The model under review builds one solid part; all positions refer to its coordinate system, in mm. Coordinates: 2 decimals unless noted, no trailing zeros. Order: outer loops, then holes, each group sorted by start corner. A loop starts at its lowest first (then second) coordinate and runs counter-clockwise, first axis right, second up. Notation, with made-up numbers: (51, -33.75) -> (57, -33.75) arc R19 cw to (57, -17.75) -> close; hole circle Ø8 at (54, 23). An arc over 180 degrees is marked (long way). Use one line per item in the form item = value. Start each with the question number.
(1) Insertion check: pin 1 Ø0.7 at (x, z) = (-83.5, 39.5) entering from +Y; pin 2 Ø0.7 at (x, y) = (-84, -368) entering from +Z; pin 3 Ø1.5 at (x, z) = (-80, 2) entering from +Y. Each pin has a flat end and moves straight along its axis. Give the tip position at first contact, or say it passes through.
(2) Take a section at B-B (x = -76). State the section outline as (y, z) points.
(3) Mouldability with a two-part tool opening along Y and no side actions: class faces 1 (the flat face through (-83.342, -369, 46)), 2 (the flat face through (-79, -369, 85)), 3 (the cylindrical face through (-72.925, -367.02, 36.835)) as +Y half, -Y half, draft (parallel to the pull), parting line (faces both ways), or undercut.
(4) Wall thickness on line 1 along X through (y, z) = (-369, 50); line 2 along Y through (x, z) = (-78.75, 67); line 3 along Y through (x, z) = (-75.5, 54.5): over which ranges is each line inside the solid? List them lowest first.
(5) Take a section at A-A (y = -373). State the section outline as (x, z) points.
```python
from build123d import *

# Parameters (mm, degrees)
BOSS_EXTRUDE1_DEPTH      = 85
BOSS_EXTRUDE1_DEPTH_BACK = 10
SKETCH1_R                = 6
SKETCH2_W                = 2.203214475
SKETCH2_H                = 4.25945658
CUT_EXTRUDE1_DEPTH       = 80


with BuildPart() as part:
    # Sketch1 → Boss-Extrude1 (new, two sides: drawn at the far end of the back side and taken through both)
    with BuildSketch(Plane.XY.offset(-BOSS_EXTRUDE1_DEPTH_BACK)):
        with Locations((-78.64751379, -368.822211525)):
            Circle(SKETCH1_R)
    extrude(amount=BOSS_EXTRUDE1_DEPTH + BOSS_EXTRUDE1_DEPTH_BACK)

    # Sketch2 → Cut-Extrude1 (cut)
    with BuildSketch(Plane.XY.offset(85)):
        with Locations((-84.444038678, -368.822211525)):
            Rectangle(SKETCH2_W, SKETCH2_H)
    extrude(amount=-CUT_EXTRUDE1_DEPTH, mode=Mode.SUBTRACT)


solid = part.part
```
Findings:
q1.pin_1 = -364.86
q1.pin_2 = 5
q1.pin_3 = -362.85
q2.outline = (-374.21, -10) -> (-363.44, -10) -> (-363.44, 85) -> (-374.21, 85) -> close
q3.face_1 = undercut
q3.face_2 = draft
q3.face_3 = parting line
q4.line_1 = -83.34 to -72.65
q4.line_2 = -374.82 to -362.82
q4.line_3 = -373.93 to -363.71
q5.outline = (-82.95, -10) -> (-74.34, -10) -> (-74.34, 85) -> (-82.95, 85) -> close
